Build history of the part. All positions in model axes, mm. Coordinates: 2 decimals unless noted, no trailing zeros. Write each loop counter-clockwise with the first axis right and the second up, starting at its lowest first coordinate (ties: lowest second). Pieces come first, ordered by that corner, then holes. Notation, with made-up numbers: (64, -6) -> (76, -6) arc R26 cw to (76, 12) -> close; hole circle Ø1 at (24.25, 41.5). An arc over 180 degrees is marked (long way). Write each question's results on one line, items separated by ' | '. Start each with the question number.
Q1. Two-plate mould, pull along X, no slides. Class faces 1 (the face through (32.468, 0.464, 0.737)), 2 (the face through (-1, 10, 0)), 3 (the face through (72, 0, 0)): released by +X, released by -X, zero draft, split by the parting line, or undercut.
Q2. Drop a flat-ended pin along its axis: pin 1 Ø6.5 at (x, y) = (-34, 0) entering from +Z. Give the stop position or say it passes through.
Q3. Drill centre lines: line 1 (Y direction, x = -34, z = -1); line 2 (X direction, y = 1, z = 2). Where is each one in solid material? Low to high.
Q4. Saw through at B-B on y = 0. Give the cut face in (x, z).
Q5. Saw through at A-A on x = -34. Give the cut face in (y, z), and give its area (3 significant figures).
Q6. Saw through at C-C on z = -1.2. Give the cut face in (x, y).
from build123d import *

# Parameters (mm, degrees)
SKETCH1_W           = 144
SKETCH1_H           = 20
BOSS_EXTRUDE1_DEPTH = 3
LPATTERN1_COUNT     = 2
LPATTERN1_PITCH     = 70


with BuildPart() as part:
    # Sketch1 → Boss-Extrude1 (new body, symmetric)
    with BuildSketch(Plane.XY):
        Rectangle(SKETCH1_W, SKETCH1_H)
    extrude(amount=BOSS_EXTRUDE1_DEPTH, both=True)

    # Sketch6 → Hole1 (revolve, cut)
    with BuildSketch(Plane(origin=(-34, 0, 3), x_dir=(0, -1, 0), z_dir=(1, 0, 0))):
        Polygon((0, 0), (0, 6), (3.5, 6), (3.5, 2.414213562), (4.5, 0), align=None)
    hole1 = revolve(axis=Axis((-34, 0, 9.445314094), (0, 0, -1)), mode=Mode.SUBTRACT)

    # LPattern1: Hole1 ×2
    with Locations(*[(i * LPATTERN1_PITCH, 0, 0) for i in range(1, LPATTERN1_COUNT)]):
        add(hole1, mode=Mode.SUBTRACT)


solid = part.part
Returned:
1) face 1: undercut | face 2: zero draft | face 3: released by +X
2) pin 1: passes through
3) line 1: y = -10 to -3.5, 3.5 to 10 | line 2: x = -72 to -37.96, -30.04 to 32.04, 39.96 to 72
4) outline: (-72, -3) -> (-37.5, -3) -> (-37.5, 0.59) -> (-38.5, 3) -> (-72, 3) -> close; (-30.5, -3) -> (32.5, -3) -> (32.5, 0.59) -> (31.5, 3) -> (-29.5, 3) -> (-30.5, 0.59) -> close; (39.5, -3) -> (72, -3) -> (72, 3) -> (40.5, 3) -> (39.5, 0.59) -> close
5) outline: (-10, -3) -> (-3.5, -3) -> (-3.5, 0.59) -> (-4.5, 3) -> (-10, 3) -> close; (3.5, -3) -> (10, -3) -> (10, 3) -> (4.5, 3) -> (3.5, 0.59) -> close | area: 75.6 mm2
6) outline: (-72, -10) -> (72, -10) -> (72, 10) -> (-72, 10) -> close; hole circle Ø7 at (-34, 0); hole circle Ø7 at (36, 0)
